from build123d import *

# Parameters (mm, degrees)
F0_W     = 76.2
F0_H     = 76.2
F1_DEPTH = 3.175
F2_W     = 76.2
F2_H     = 73.025
F3_DEPTH = 3.175
F2_H_2   = 76.2
F4_DEPTH = 3.175
F5_W     = 76.2
F5_H     = 76.2
F6_DEPTH = 3.175


# Not quite as in the source:
# - a length typed as a fraction of an inch, garbled in the dataset ("3 / 203.2 mm" for 3/8 in), is restored


with BuildPart() as f1:
    # F0 (on Top) → F1 (new body)
    with BuildSketch(Plane.XY):
        Rectangle(F0_W, F0_H)
    extrude(amount=F1_DEPTH)

    # F2 (on face) → F3 (join)
    with BuildSketch(Plane.XZ.offset(38.1)):
        with Locations((0, 39.6875)):
            Rectangle(F2_W, F2_H)
    extrude(amount=F3_DEPTH)

    # F2 (on face) → F4 (join)
    with BuildSketch(Plane.XZ.offset(38.1)):
        with Locations((0, 38.1)):
            Rectangle(F2_W, F2_H_2)
    extrude(amount=F4_DEPTH)

    # F5 (on face) → F6 (join)
    with BuildSketch(Plane(origin=(0, 38.1, 0), x_dir=(-1, 0, 0), z_dir=(0, 1, 0))):
        with Locations((0, 38.1)):
            Rectangle(F5_W, F5_H)
    extrude(amount=F6_DEPTH)


solid = f1.part
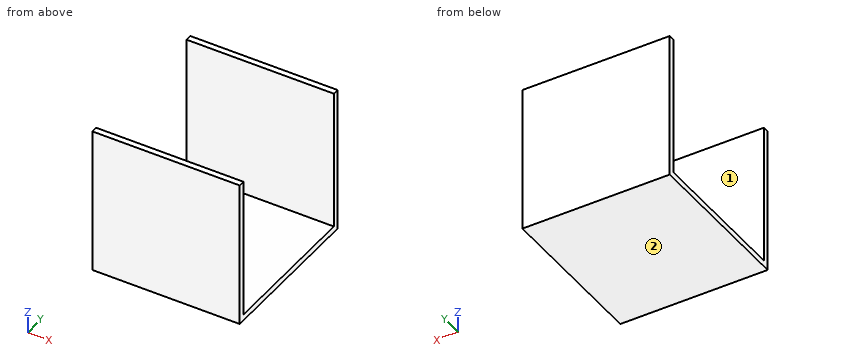
Geometry check sheet. Reference: the model listing, model coordinates, mm. Face numbers are marked on the shaded views. A direction names the side the tool comes from. Round coordinates to 2 decimals unless told otherwise and drop trailing zeros. Order: outer loops, then holes, each group sorted by start corner. A loop starts at its lowest first (then second) coordinate and runs counter-clockwise, first axis right, second up. Notation, with made-up numbers: (89.25, 30) - (146.25, 30) arc R33 ccw to (146.25, 61) - close; hole circle Ø9 at (-5.75, 59). An arc over 180 degrees is marked (long way). One line per question, with ' | ' between items. Start each with the question number.
(1) Sectioned sample at B-B on x = 3. Record the cut outline in (y, z) (3 decimals).
(2) Depth check by flat-ended pin: pin 1 Ø1.5 at (x, y) = (18, -21.5) entering from +Z (3 decimals). Enter the tip coordinate at first touch or a pass-through.
(3) Access from +Z, -Z, +X, -X, +Y, -Y to the whole of each face (thin tool, end or side, straight path). Record for the marked faces 1 and 2.
(4) Sectioned sample at A-A on z = 35. Record the cut outline in (x, y) (3 decimals).
(5) Thickness scan on L1, parallel to Y at x = -5.5, z = 72 (3 decimals); L2, parallel to Z at x = -5.5, y = -24 (3 decimals). Record the ranges inside material, lowest first. Write a range as [from, to].
(6) Sectioned sample at C-C on y = -5. Record the cut outline in (x, z) (3 decimals), and give its area (3 significant figures).
Conclusion:
1) outline: (-41.275, 0) - (41.275, 0) - (41.275, 76.2) - (38.1, 76.2) - (38.1, 3.175) - (-38.1, 3.175) - (-38.1, 76.2) - (-41.275, 76.2) - close
2) pin 1: stops at z = 3.175
3) face 1: +Z, +X, -X | face 2: -Z, +X, -X, +Y, -Y
4) outline: (-38.1, -41.275) - (38.1, -41.275) - (38.1, -38.1) - (-38.1, -38.1) - close; (-38.1, 38.1) - (38.1, 38.1) - (38.1, 41.275) - (-38.1, 41.275) - close
5) L1: y = [-41.275, -38.1], [38.1, 41.275] | L2: z = [0, 3.175]
6) outline: (-38.1, 0) - (38.1, 0) - (38.1, 3.175) - (-38.1, 3.175) - close | area: 242 mm2
